Source: CAD feature listing. Evaluate the final solid. Frame: model axes, mm. A direction names the side the tool comes from. Round coordinates to 2 decimals unless told otherwise and drop trailing zeros. Order: outer loops, then holes, each group sorted by start corner. A loop starts at its lowest first (then second) coordinate and runs counter-clockwise, first axis right, second up. Notation, with made-up numbers: (77.25, 8.5) -> (116.25, 8.5) arc R12 cw to (116.25, 20.5) -> close; hole circle Ø7 at (55, 85). An arc over 180 degrees is marked (long way). One line per item, written item: value. Start each with the question number.
1) Ray query, L1, parallel to Z at x = 17, y = 5; L2, parallel to X at y = 12, z = 0.75; L3, parallel to Y at x = 30.5, z = -10.25. Return the intervals inside material, ascending.
2) Section C-C (x = 24.5). Return the cut outline in (y, z), and give its area (3 significant figures).
3) Section B-B (y = 31). Return the cut outline in (x, z), and give its area (3 significant figures).
4) Section A-A (x = 51). Return the cut outline in (y, z), and give its area (3 significant figures).
5) Reachability of faces 4 (the face through (2.281, 52.594, 2.535)), 5 (the face through (41.5, 29, 3)), 6 (the face through (9.1, 12.5, 2.5)) from +Z, -Z, +X, -X, +Y, -Y: full face, straight path, thin tool, end or side. Return the list, or none.
6) Mould query, pull axis X, two halves, no side actions, for faces 1 (the face through (43, 31, 0)), 2 (the face through (48.5, 30, 3)), 3 (the face through (57.719, 52.594, 2.535)). Classes: pulls with the +X half, pulls with the -X half, needs draft (parallel to the pull), parting line crosses it, or undercut.
7) Pin query (flat end, axial travel): P1, Ø1.5, axis at x = 31, z = 1.5, coming from the +Y side; P2, Ø8, axis at x = 43, z = -5, coming from the -Y side; P3, Ø24, axis at x = 43.5, y = 27, coming from the -Z side; P4, Ø5, axis at x = 40.5, z = 0.5, coming from the +Y side. Return the tip coordinate at first contact, or that it passes through.
8) Section D-D (z = 1.5). Return the cut outline in (x, y).
```python
from build123d import *

# Parameters (mm, degrees)
SKETCH1_W           = 60
SKETCH1_H           = 55
BOSS_EXTRUDE1_DEPTH = 5
CUT_EXTRUDE1_REACH  = 83.548
SKETCH2_W           = 23
SKETCH2_H           = 44
SKETCH3_W           = 60
SKETCH3_H           = 7
BOSS_EXTRUDE2_DEPTH = 15
CUT_EXTRUDE2_REACH  = 80.288
SKETCH4_R           = 2.5
FILLET1_R           = 8
FILLET2_R           = 5
FILLET3_R           = 5
FILLET4_R           = 1


with BuildPart() as part:
    # Sketch1 → Boss-Extrude1 (new body)
    with BuildSketch(Plane.XY):
        with Locations((30, 27.5)):
            Rectangle(SKETCH1_W, SKETCH1_H)
    extrude(amount=BOSS_EXTRUDE1_DEPTH)

    # Sketch2 → Cut-Extrude1 (cut, up to next)
    with BuildSketch(Plane.XY.offset(5), mode=Mode.PRIVATE) as cut_extrude1_sk1:
        with BuildLine():
            Line((11.5, 45), (11.5, 15))
            ThreePointArc((11.5, 15), (9, 12.5), (6.5, 15))
            Line((6.5, 15), (6.5, 45))
            ThreePointArc((6.5, 45), (9, 47.5), (11.5, 45))
        make_face()
    cut_extrude1_tool1 = extrude(cut_extrude1_sk1.sketch, amount=-CUT_EXTRUDE1_REACH, mode=Mode.PRIVATE) & part.part
    # Sketch2 → Cut-Extrude1 (cut, up to next)
    with BuildSketch(Plane.XY.offset(5), mode=Mode.PRIVATE) as cut_extrude1_sk2:
        with BuildLine():
            Line((53.5, 45), (53.5, 15))
            ThreePointArc((53.5, 15), (51, 12.5), (48.5, 15))
            Line((48.5, 15), (48.5, 45))
            ThreePointArc((48.5, 45), (51, 47.5), (53.5, 45))
        make_face()
    cut_extrude1_tool2 = extrude(cut_extrude1_sk2.sketch, amount=-CUT_EXTRUDE1_REACH, mode=Mode.PRIVATE) & part.part
    # Sketch2 → Cut-Extrude1 (cut, up to next)
    with BuildSketch(Plane.XY.offset(5), mode=Mode.PRIVATE) as cut_extrude1_sk3:
        with Locations((30, 33)):
            Rectangle(SKETCH2_W, SKETCH2_H)
    cut_extrude1_tool3 = extrude(cut_extrude1_sk3.sketch, amount=-CUT_EXTRUDE1_REACH, mode=Mode.PRIVATE) & part.part
    add(cut_extrude1_tool1.solids().sort_by_distance((9, 30, 5))[0], mode=Mode.SUBTRACT)
    add(cut_extrude1_tool2.solids().sort_by_distance((51, 30, 5))[0], mode=Mode.SUBTRACT)
    add(cut_extrude1_tool3.solids().sort_by_distance((30, 33, 5))[0], mode=Mode.SUBTRACT)

    # Sketch3 → Boss-Extrude2 (add)
    with BuildSketch(Plane(origin=(0, 0, 0), x_dir=(-1, 0, 0), z_dir=(0, 0, -1))):
        with Locations((-30, 3.5)):
            Rectangle(SKETCH3_W, SKETCH3_H)
    extrude(amount=BOSS_EXTRUDE2_DEPTH)

    # Sketch4 → Cut-Extrude2 (cut, up to next)
    with BuildSketch(Plane(origin=(0, 7, 0), x_dir=(1, 0, 0), z_dir=(0, 1, 0)), mode=Mode.PRIVATE) as cut_extrude2_sk1:
        with Locations(Location((17, 5, 0), (0, 0, 180))):
            Circle(SKETCH4_R)
    cut_extrude2_tool1 = extrude(cut_extrude2_sk1.sketch, amount=-CUT_EXTRUDE2_REACH, mode=Mode.PRIVATE) & part.part
    # Sketch4 → Cut-Extrude2 (cut, up to next)
    with BuildSketch(Plane(origin=(0, 7, 0), x_dir=(1, 0, 0), z_dir=(0, 1, 0)), mode=Mode.PRIVATE) as cut_extrude2_sk2:
        with Locations(Location((43, 5, 0), (0, 0, 180))):
            Circle(SKETCH4_R)
    cut_extrude2_tool2 = extrude(cut_extrude2_sk2.sketch, amount=-CUT_EXTRUDE2_REACH, mode=Mode.PRIVATE) & part.part
    add(cut_extrude2_tool1.solids().sort_by_distance((17, 7, -5))[0], mode=Mode.SUBTRACT)
    add(cut_extrude2_tool2.solids().sort_by_distance((43, 7, -5))[0], mode=Mode.SUBTRACT)

    # Fillet1
    fillet1_edges = [part.edges().sort_by_distance(p)[0] for p in [
        (18.5, 55, 2.5),
        (41.5, 55, 2.5),
        (0, 55, 2.5),
        (60, 55, 2.5),
    ]]
    fillet(fillet1_edges, radius=FILLET1_R)

    # Fillet2
    fillet2_edges = [part.edges().sort_by_distance(p)[0] for p in [
        (0, 3.5, -15),
        (60, 3.5, -15),
    ]]
    fillet(fillet2_edges, radius=FILLET2_R)

    # Fillet3
    fillet3_edges = [part.edges().sort_by_distance(p)[0] for p in [
        (30, 0, 5),
    ]]
    fillet(fillet3_edges, radius=FILLET3_R)

    # Fillet4
    fillet4_edges = [part.edges().sort_by_distance(p)[0] for p in [
        (18.5, 11, 2.5),
        (41.5, 11, 2.5),
    ]]
    fillet(fillet4_edges, radius=FILLET4_R)


solid = part.part
```
Findings:
1. L1: -15 to -7.5, -2.5 to 5
1. L2: 0 to 18.5, 41.5 to 60
1. L3: 0 to 7
2. outline: (0, -15) -> (7, -15) -> (7, 0) -> (11, 0) -> (11, 5) -> (5, 5) arc R5 ccw to (0, 0) -> close
2. area: 155 mm2
3. outline: (0, 0) -> (6.5, 0) -> (6.5, 5) -> (0, 5) -> close; (11.5, 0) -> (18.5, 0) -> (18.5, 5) -> (11.5, 5) -> close; (41.5, 0) -> (48.5, 0) -> (48.5, 5) -> (41.5, 5) -> close; (53.5, 0) -> (60, 0) -> (60, 5) -> (53.5, 5) -> close
3. area: 135 mm2
4. outline: (0, -15) -> (7, -15) -> (7, 0) -> (12.5, 0) -> (12.5, 5) -> (5, 5) arc R5 ccw to (0, 0) -> close; (47.5, 0) -> (55, 0) -> (55, 5) -> (47.5, 5) -> close
4. area: 200 mm2
5. face 4: +Z, -Z, -X, +Y
5. face 5: +Z, -Z, +Y
5. face 6: +Z, -Z
6. face 1: needs draft
6. face 2: undercut
6. face 3: pulls with the +X half
7. P1: y = 11
7. P2: y = 0
7. P3: z = 0
7. P4: y = 51.66
8. outline: (0, 0.23) -> (60, 0.23) -> (60, 47) arc R8 ccw to (52, 55) -> (49.5, 55) arc R8 ccw to (41.5, 47) -> (41.5, 12) arc R1 cw to (40.5, 11) -> (19.5, 11) arc R1 cw to (18.5, 12) -> (18.5, 47) arc R8 ccw to (10.5, 55) -> (8, 55) arc R8 ccw to (0, 47) -> close; hole (6.5, 15) arc R2.5 ccw to (11.5, 15) -> (11.5, 45) arc R2.5 ccw to (6.5, 45) -> close; hole (48.5, 15) arc R2.5 ccw to (53.5, 15) -> (53.5, 45) arc R2.5 ccw to (48.5, 45) -> close
